from build123d import *

# Parameters (mm, degrees)
SKETCH1_R               = 3
BOSS_EXTRUDE1_DEPTH     = 97
SKETCH2_R               = 4
BOSS_EXTRUDE2_DEPTH     = 4.7
SKETCH3_R               = 9
BOSS_EXTRUDE3_DEPTH     = 7.9
SKETCH4_R               = 5.9
BOSS_EXTRUDE4_DEPTH     = 8
SKETCH5_R               = 9
BOSS_EXTRUDE5_DEPTH     = 3
SKETCH6_R               = 1.4
CUT_EXTRUDE1_DEPTH      = 82
CUT_EXTRUDE1_DEPTH_BACK = 82
SKETCH7_R               = 3
SKETCH7_R_2             = 0.75
CUT_EXTRUDE2_DEPTH      = 9


with BuildPart() as part:
    # Sketch1 → Boss-Extrude1 (new body)
    with BuildSketch(Plane.XY):
        Circle(SKETCH1_R)
    extrude(amount=BOSS_EXTRUDE1_DEPTH)

    # Sketch2 → Boss-Extrude2 (add)
    with BuildSketch(Plane.XY.offset(97)):
        Circle(SKETCH2_R)
    extrude(amount=BOSS_EXTRUDE2_DEPTH)

    # Sketch3 → Boss-Extrude3 (add)
    with BuildSketch(Plane.XY.offset(101.7)):
        Circle(SKETCH3_R)
    extrude(amount=BOSS_EXTRUDE3_DEPTH)

    # Sketch4 → Boss-Extrude4 (add)
    with BuildSketch(Plane.XY.offset(109.6)):
        Circle(SKETCH4_R)
    extrude(amount=BOSS_EXTRUDE4_DEPTH)

    # Sketch5 → Boss-Extrude5 (add)
    with BuildSketch(Plane.XY.offset(117.6)):
        Circle(SKETCH5_R)
    extrude(amount=BOSS_EXTRUDE5_DEPTH)

    # Sketch6 → Cut-Extrude1 (cut, two sides)
    with BuildSketch(Plane(origin=(0, 0, 0), x_dir=(1, 0, 0), z_dir=(0, 1, 0))) as cut_extrude1_sk:
        with Locations((0, -38.9)):
            Circle(SKETCH6_R)
    extrude(amount=CUT_EXTRUDE1_DEPTH, mode=Mode.SUBTRACT)
    extrude(cut_extrude1_sk.sketch, amount=-CUT_EXTRUDE1_DEPTH_BACK, mode=Mode.SUBTRACT)

    # Sketch7 → Cut-Extrude2 (cut)
    with BuildSketch(Plane.XY.offset(120.6)):
        Circle(SKETCH7_R)
        with Locations((1.637751338, 7.588247864)):
            Circle(SKETCH7_R_2)
    extrude(amount=-CUT_EXTRUDE2_DEPTH, mode=Mode.SUBTRACT)


solid = part.part
Verification items for the finished model (mm, model axes). A direction names the side the tool comes from. Give positions to 0.01 mm unless a question says otherwise; leave off trailing zeros. Loops run counter-clockwise (first coordinate to the right, second up) from the corner with the lowest first, then second, coordinate; pieces in that order, holes last.
1. Cross-section at B-B on y = -7.25. Record the cut outline in (x, z), and give its area (3 significant figures).
Derived:
outline: (-5.33, 101.7) - (5.33, 101.7) - (5.33, 109.6) - (-5.33, 109.6) - close; (-5.33, 117.6) - (5.33, 117.6) - (5.33, 120.6) - (-5.33, 120.6) - close
area: 116 mm2
2. Cross-section at D-D on z = 38.9. Record the cut outline in (x, y), and give its area (3 significant figures).
Derived:
outline: (-1.4, -2.65) - (-1.4, 2.65) arc R3 ccw to start; (1.4, -2.65) arc R3 ccw to (1.4, 2.65) - close
area: 12.1 mm2
3. Go/stop test with flat-tipped pins: P1, Ø1, axis at y = -4.5, z = 107.5, coming from the -X side; P2, Ø8, axis at x = -6, z = 46, coming from the +Y side; P3, Ø3.5, axis at x = 0, z = 38.9, coming from the -Y side. Record where each tip stops, or that it passes through.
Derived:
P1: stops at x = -8.06
P2: stops at y = 2.24
P3: stops at y = -3
4. Cross-section at A-A on x = -7.5. Record the cut outline in (y, z).
Derived:
outline: (-4.97, 101.7) - (4.97, 101.7) - (4.97, 109.6) - (-4.97, 109.6) - close; (-4.97, 117.6) - (4.97, 117.6) - (4.97, 120.6) - (-4.97, 120.6) - close
5. Cross-section at C-C on z = 63.5. Record the cut outline in (x, y).
Derived:
outline: circle Ø6 at (0, 0)
6. Release check for a two-part mould opening along X. For faces 1 (the cylindrical face through (-3, 0, 116)), 2 (the cylindrical face through (-3, 0, 48)), 3 (the flat face through (2, -6, 117.6)) record: +X half, -X half, draft (parallel to the pull), parting line (faces both ways), or undercut.
Derived:
face 1: undercut
face 2: parting line
face 3: draft
7. Material ranges on probe 1 along Z at (x, y) = (-5.75, 2); probe 2 along Z at (x, y) = (0, -1.5); probe 3 along Y at (x, z) = (0, 118.25), recorded low to high.
Derived:
probe 1: z = 101.7 to 109.6, 117.6 to 120.6
probe 2: z = 0 to 37.5, 40.3 to 111.6
probe 3: y = -9 to -3, 3 to 9
8. Tool access check on faces 4 (the flat face through (1, 3, 97)), 5 (the flat face through (0, 0, 111.6)), 6 (the flat face through (2, -6, 109.6)), 7 (the cylindrical face through (-1.172, 8.923, 119.079)). Record the directions out of +Z, -Z, +X, -X, +Y, -Y that give a thin tool (end or side, any length) a straight path to the whole face; none if there is none.
Derived:
face 4: -Z
face 5: +Z
face 6: none
face 7: +Z, -Z
